Job drawing, mm, ordinate dimensions from the low corner. One solid piece. A direction names the side the tool comes from. Round coordinates to 2 decimals unless told otherwise and drop trailing zeros. Write each loop counter-clockwise with the first axis right and the second up, starting at its lowest first coordinate (ties: lowest second). Pieces come first, ordered by that corner, then holes. Notation, with made-up numbers: (4.5, 66) -> (60.5, 66) arc R23 cw to (60.5, 85) -> close; hole circle Ø6 at (60.5, 9.5). An arc over 180 degrees is marked (long way). Use CSV: the item, a comma, the result in double quotes. Start each with the question number.
(1) Drop flat-ended pins along their axis: pin 1 (2.5 mm diameter, centred on y = 5, z = 35, fed in from +X); pin 2 (1 mm diameter, centred on x = 8, z = 30, fed in from +Y); pin 3 (2.5 mm diameter, centred on y = 5.5, z = 15.5, fed in from +X). Give the stop position or say it passes through.
(2) Saw through at A-A (y = 5). Give the cut face in (x, z).
(3) Probe line 1 (Z direction, x = 0.6, y = 5); line 2 (Y direction, x = 0.2, z = 35); line 3 (Z direction, x = 0.75, y = 4). List the from-to ranges inside material, lowest first. Write a range as [from, to].
(4) Saw through at B-B (z = 5). Give the cut face in (x, y), plus the area to 3 significant figures.
(5) Saw through at D-D (x = 4.5). Give the cut face in (y, z), plus the area to 3 significant figures.
(6) Which spindle directions (+Z, -Z, +X, -X, +Y, -Y) get a long thin tool onto all of the face, cutting with end or side? Do the marked faces 1 and 2. Say none if no direction does.
(7) Saw through at C-C (z = 14). Give the cut face in (x, y).
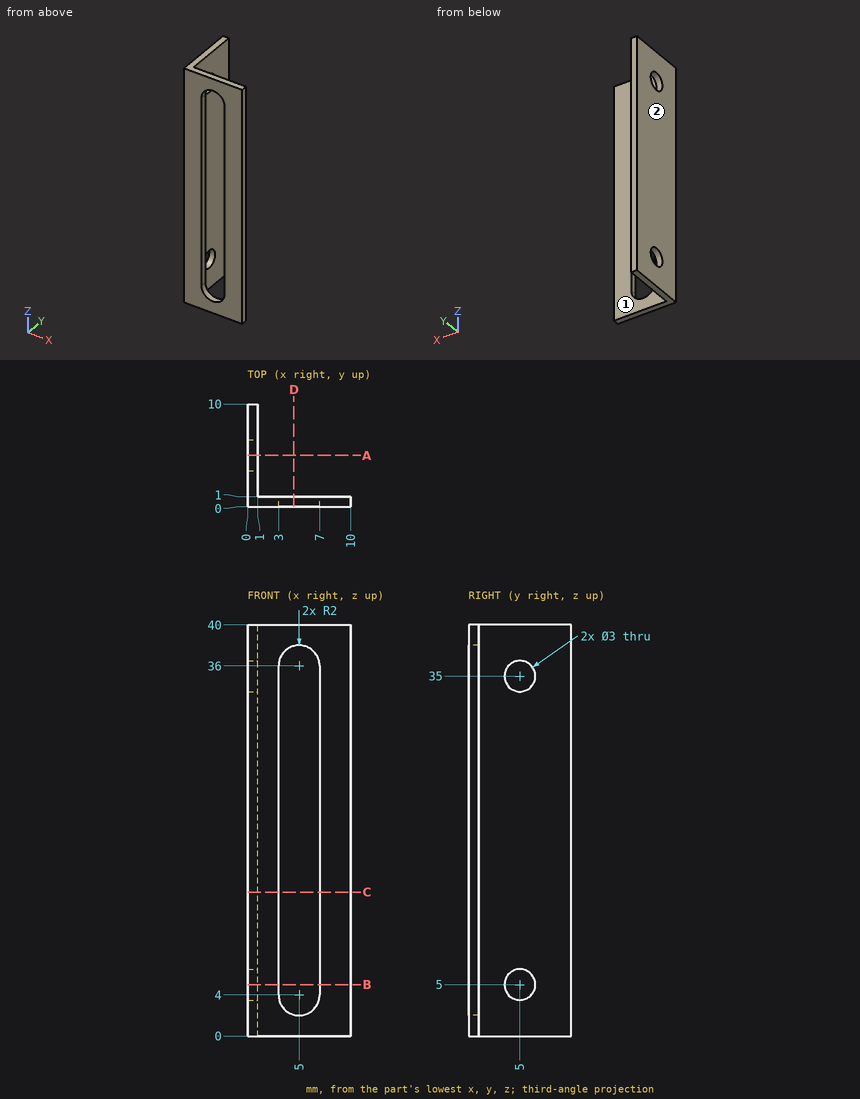
Answers:
1,pin 1,"passes through"
1,pin 2,"stops at y = 1"
1,pin 3,"stops at x = 1"
2,outline,"(0, 0) -> (1, 0) -> (1, 3.5) -> (0, 3.5) -> close; (0, 6.5) -> (1, 6.5) -> (1, 33.5) -> (0, 33.5) -> close; (0, 36.5) -> (1, 36.5) -> (1, 40) -> (0, 40) -> close"
3,line 1,"z = [0, 3.5], [6.5, 33.5], [36.5, 40]"
3,line 2,"y = [0, 3.5], [6.5, 10]"
3,line 3,"z = [0, 3.88], [6.12, 33.88], [36.12, 40]"
4,outline,"(0, 0) -> (3, 0) -> (3, 1) -> (1, 1) -> (1, 3.5) -> (0, 3.5) -> close; (0, 6.5) -> (1, 6.5) -> (1, 10) -> (0, 10) -> close; (7, 0) -> (10, 0) -> (10, 1) -> (7, 1) -> close"
4,area,"12.0 mm²"
5,outline,"(0, 0) -> (1, 0) -> (1, 2.06) -> (0, 2.06) -> close; (0, 37.94) -> (1, 37.94) -> (1, 40) -> (0, 40) -> close"
5,area,"4.13 mm²"
6,face 1,"+Z, -Z, +X, +Y"
6,face 2,"+Z, -Z, -X, +Y, -Y"
7,outline,"(0, 0) -> (3, 0) -> (3, 1) -> (1, 1) -> (1, 10) -> (0, 10) -> close; (7, 0) -> (10, 0) -> (10, 1) -> (7, 1) -> close"
